For this review, take the finished solid that the model builds, in its own axes (mm). Coordinates: 2 decimals unless noted, no trailing zeros. Loops run counter-clockwise (first coordinate to the right, second up) from the corner with the lowest first, then second, coordinate; pieces in that order, holes last. Notation, with made-up numbers: (26.25, -11) - (39.25, -11) arc R35 ccw to (39.25, 26) - close; hole circle Ø2 at (62.25, 9.25). An arc over 180 degrees is marked (long way). Use one line per item in the form item = value. Start each with the question number.
1. Add section A-A on z = 19.05. Give the boundary of the cut face in (x, y), and give its area (3 significant figures).
2. Add section B-B on y = 4.75. Give the boundary of the cut face in (x, z).
3. Draft analysis for pull direction X (two halves, no side actions). For faces 1 (the face through (247.08, 3.22, -12.76)), 2 (the face through (-74, 6.35, -2)), state which applies: +X half, -X half, draft (parallel to the pull), parting line (faces both ways), or undercut.
4. Add section C-C on x = 146.05. Give the boundary of the cut face in (y, z), and give its area (3 significant figures).
5. To check wall thickness, follow probe 1 along X at (y, z) = (0.5, -111); probe 2 along Z at (x, y) = (146.05, 3.5); probe 3 along X at (y, z) = (2.5, 19.05). State the ranges of each line that lie inside material, in increasing order.
6. For pin 1 Ø1.1 at (x, y) = (306.5, 4.5) entering from +Z (3 decimals); pin 2 Ø3 at (x, y) = (-307, 4.5) entering from +Z, all flat-tipped, find the tip position at first contact; note any pin that passes through.
```python
from build123d import *

# Parameters (mm, degrees)
CROQUIS2_W              = 622.3
CROQUIS2_H              = 304.8
SALIENTE_EXTRUIR1_DEPTH = 6.35
REDONDEO1_R             = 6.35
CROQUIS4_W              = 3.81
CROQUIS4_H              = 76.2
CORTAR_EXTRUIR2_DEPTH   = 7.35
CROQUIS5_R              = 105.918
CORTAR_EXTRUIR3_DEPTH   = 7.35


with BuildPart() as part:
    # Croquis2 → Saliente-Extruir1 (new body)
    with BuildSketch(Plane(origin=(0, 0, 0), x_dir=(1, 0, 0), z_dir=(0, 1, 0))):
        Rectangle(CROQUIS2_W, CROQUIS2_H)
    extrude(amount=SALIENTE_EXTRUIR1_DEPTH)

    # Redondeo1
    redondeo1_edges = [part.edges().sort_by_distance(p)[0] for p in [
        (311.15, 3.175, 152.4),
        (-311.15, 3.175, 152.4),
    ]]
    fillet(redondeo1_edges, radius=REDONDEO1_R)

    # Croquis4 → Cortar-Extruir2 (cut, through all)
    with BuildSketch(Plane(origin=(0, 6.35, 0), x_dir=(1, 0, 0), z_dir=(0, 1, 0))):
        with Locations((-306.705, 101.6)):
            Rectangle(CROQUIS4_W, CROQUIS4_H)
        with Locations((306.705, 101.6)):
            Rectangle(CROQUIS4_W, CROQUIS4_H)
    extrude(amount=-CORTAR_EXTRUIR2_DEPTH, mode=Mode.SUBTRACT)

    # Croquis5 → Cortar-Extruir3 (cut, through all)
    with BuildSketch(Plane(origin=(0, 6.35, 0), x_dir=(1, 0, 0), z_dir=(0, 1, 0))):
        with Locations((146.05, -19.05)):
            Circle(CROQUIS5_R)
    extrude(amount=-CORTAR_EXTRUIR3_DEPTH, mode=Mode.SUBTRACT)


solid = part.part
```
Conclusion:
q1.outline = (-311.15, 0) - (40.13, 0) - (40.13, 6.35) - (-311.15, 6.35) - close; (251.97, 0) - (311.15, 0) - (311.15, 6.35) - (251.97, 6.35) - close
q1.area = 2,610 mm^2
q2.outline = (-311.15, -152.4) - (311.15, -152.4) - (311.15, 146.05) arc R6.35 ccw to (304.8, 152.4) - (-304.8, 152.4) arc R6.35 ccw to (-311.15, 146.05) - close; hole (-308.61, -139.7) - (-304.8, -139.7) - (-304.8, -63.5) - (-308.61, -63.5) - close; hole circle Ø211.84 at (146.05, 19.05); hole (304.8, -139.7) - (308.61, -139.7) - (308.61, -63.5) - (304.8, -63.5) - close
q3.face_1 = undercut
q3.face_2 = draft
q4.outline = (0, -152.4) - (6.35, -152.4) - (6.35, -86.87) - (0, -86.87) - close; (0, 124.97) - (6.35, 124.97) - (6.35, 152.4) - (0, 152.4) - close
q4.area = 590 mm^2
q5.probe_1 = -311.15 to -308.61, -304.8 to 304.8, 308.61 to 311.15
q5.probe_2 = -152.4 to -86.87, 124.97 to 152.4
q5.probe_3 = -311.15 to 40.13, 251.97 to 311.15
q6.pin_1 = 152.295
q6.pin_2 = 152.36
